Could you check a few things on this model? Use its own coordinates, in mm. Coordinates: 2 decimals unless noted, no trailing zeros.
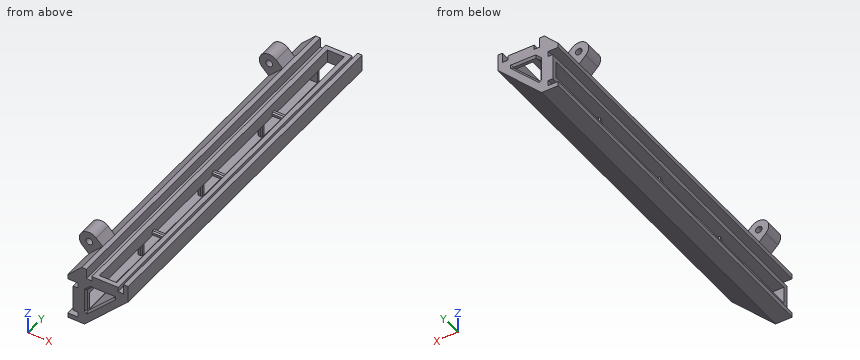
from build123d import *

# Parameters (mm, degrees)
BOSS_EXTRUDE4_DEPTH      = 247.65
CUT_EXTRUDE9_DEPTH       = 247.65
SKETCH11_W               = 11.65
SKETCH11_H               = 241.3
CUT_EXTRUDE7_DEPTH       = 9.017
SKETCH12_W               = 11.65
SKETCH12_H               = 241.3
CUT_EXTRUDE8_DEPTH       = 9.017
SKETCH16_R               = 2.286
BOSS_EXTRUDE5_DEPTH      = 12.7
CHAMFER1_SIZE            = 0.493914087
CHAMFER1_SIZE_2          = 0.6985
CHAMFER2_SIZE            = 3.175
CHAMFER3_SIZE            = 1.27
BOSS_EXTRUDE6_DEPTH      = 1.5875
BOSS_EXTRUDE6_DEPTH_BACK = 1.5875
SKETCH19_W               = 11.65
SKETCH19_H               = 3.175
SKETCH19_W_2             = 3.175
SKETCH19_H_2             = 11.4765
SKETCH20_W               = 3.175
SKETCH20_H               = 11.4765
SKETCH20_W_2             = 11.65
SKETCH20_H_2             = 3.175
BOSS_EXTRUDE7_DEPTH      = 3.175
CHAMFER4_SIZE            = 0.79375


with BuildPart() as part:
    # Sketch1 → Boss-Extrude4 (new body)
    with BuildSketch(Plane(origin=(0, 0, 0), x_dir=(1, 0, 0), z_dir=(0, 1, 0))):
        Polygon((41.275, 0), (41.275, 11.384871939), (11.384871939, 41.275), (0, 41.275), (0, 38.1), (6.858, 38.1), (6.858, 34.4), (3.683, 34.4), (3.683, 16.4), (6.858, 16.4), (6.858, 12.7), (0, 12.7), (0, 9.525), (9.525, 0), (12.7, 0), (12.7, 6.858), (16.4, 6.858), (16.4, 3.683), (34.4, 3.683), (34.4, 6.858), (38.1, 6.858), (38.1, 0), align=None)
    extrude(amount=BOSS_EXTRUDE4_DEPTH)

    # Sketch13 → Cut-Extrude9 (cut)
    with BuildSketch(Plane.XZ):
        Polygon((12.7, -12.7), (12.7, -31.75), (31.75, -12.7), align=None)
    extrude(amount=-CUT_EXTRUDE9_DEPTH, mode=Mode.SUBTRACT)

    # Sketch11 → Cut-Extrude7 (cut)
    with BuildSketch(Plane.ZY.offset(-3.683)):
        with Locations((-25.4, 123.825)):
            Rectangle(SKETCH11_W, SKETCH11_H)
    extrude(amount=-CUT_EXTRUDE7_DEPTH, mode=Mode.SUBTRACT)

    # Sketch12 → Cut-Extrude8 (cut)
    with BuildSketch(Plane.XY.offset(-3.683)):
        with Locations((25.4, 123.825)):
            Rectangle(SKETCH12_W, SKETCH12_H)
    extrude(amount=-CUT_EXTRUDE8_DEPTH, mode=Mode.SUBTRACT)

    # Sketch16 → Boss-Extrude5 (add)
    with BuildSketch(Plane(origin=(0, 225.425, 0), x_dir=(1, 0, 0), z_dir=(0, 1, 0))):
        with BuildLine():
            Line((5.034871939, -4.490128061), (9.525, 0))
            Line((9.525, 0), (0, 9.525))
            Line((0, 9.525), (-4.490128061, 5.034871939))
            ThreePointArc((-4.490128061, 5.034871939), (-4.490128061, -4.490128061), (5.034871939, -4.490128061))
        make_face()
        with Locations(Location((0.272371939, 0.272371939, 0), (0, 0, 270))):
            Circle(SKETCH16_R, mode=Mode.SUBTRACT)
    boss_extrude5 = extrude(amount=-BOSS_EXTRUDE5_DEPTH)

    # Mirror1: Boss-Extrude5 across plane
    add(boss_extrude5.mirror(Plane.ZX.offset(123.825)))

    # Chamfer1
    # the kernel refuses this chamfer: 0.6985, 0.493914087 mm, written as the material it adds along each edge
    with BuildSketch(Plane(origin=(31.75, 0, -12.7), x_dir=(-0.9984038297885895, 0, 0.056478249472492296), z_dir=(0, 1, 0))) as chamfer1_piece_1:
        Polygon((CHAMFER1_SIZE * 0.998403829099, -CHAMFER1_SIZE * 0.0564782494335), (CHAMFER1_SIZE_2 * 0.666041965215, -CHAMFER1_SIZE_2 * 0.745914271598), (0, 0), align=None)
    extrude(amount=247.65)
    with BuildSketch(Plane(origin=(12.7, 0, -31.75), x_dir=(0.745914271597676, 0, 0.6660419652145867), z_dir=(0, 1, 0))) as chamfer1_piece_2_section:
        Polygon((CHAMFER1_SIZE * 0.998403829099, -CHAMFER1_SIZE * 0.0564782494335), (CHAMFER1_SIZE_2 * 0.666041965215, -CHAMFER1_SIZE_2 * 0.745914271598), (0, 0), align=None)
    chamfer1_piece_2 = extrude(amount=247.65, mode=Mode.PRIVATE)
    chamfer1_piece_2 = split(chamfer1_piece_2, bisect_by=Plane(origin=(12.824663098, 1.5875, -31.225), z_dir=(0, 0, -1)), keep=Keep.TOP, mode=Mode.PRIVATE)
    add(chamfer1_piece_2)
    with BuildSketch(Plane(origin=(12.7, 0, -31.75), x_dir=(0.745914271597676, 0, 0.6660419652145867), z_dir=(0, 1, 0))) as chamfer1_piece_3_section:
        Polygon((CHAMFER1_SIZE * 0.998403829099, -CHAMFER1_SIZE * 0.0564782494335), (CHAMFER1_SIZE_2 * 0.666041965215, -CHAMFER1_SIZE_2 * 0.745914271598), (0, 0), align=None)
    chamfer1_piece_3 = extrude(amount=249.446320567, mode=Mode.PRIVATE)
    chamfer1_piece_3 = split(chamfer1_piece_3, bisect_by=Plane(origin=(12.757833333, 3.175, -31.167166667), z_dir=(0, -1, 0)), keep=Keep.TOP, mode=Mode.PRIVATE)
    add(chamfer1_piece_3)
    with BuildSketch(Plane(origin=(12.7, -1.796320567, -31.75), x_dir=(0.745914271597676, 0, 0.6660419652145867), z_dir=(0, 1, 0))) as chamfer1_piece_4_section:
        Polygon((CHAMFER1_SIZE * 0.998403829099, -CHAMFER1_SIZE * 0.0564782494335), (CHAMFER1_SIZE_2 * 0.666041965215, -CHAMFER1_SIZE_2 * 0.745914271598), (0, 0), align=None)
    chamfer1_piece_4 = extrude(amount=249.446320567, mode=Mode.PRIVATE)
    chamfer1_piece_4 = split(chamfer1_piece_4, bisect_by=Plane(origin=(12.757833333, 244.475, -31.167166667), z_dir=(0, 1, 0)), keep=Keep.TOP, mode=Mode.PRIVATE)
    add(chamfer1_piece_4)

    # Chamfer2
    chamfer2_edges = [part.edges().sort_by_distance(p)[0] for p in [
        (12.7, 123.825, -12.7),
    ]]
    chamfer(chamfer2_edges, length=CHAMFER2_SIZE)

    # Chamfer3
    chamfer3_edges = [part.edges().sort_by_distance(p)[0] for p in [
        (22.152667957, 0, -22.297332043),
        (22.152667957, 247.65, -22.297332043),
        (23.565542957, 0, -12.7),
        (23.565542957, 247.65, -12.7),
        (12.874625, 0, -31.226125),
        (12.874625, 247.65, -31.226125),
        (31.256085913, 0, -12.946957043),
        (31.256085913, 247.65, -12.946957043),
        (12.7, 0, -23.46325),
        (12.7, 247.65, -23.46325),
        (14.2875, 0, -14.2875),
        (14.2875, 247.65, -14.2875),
    ]]
    chamfer(chamfer3_edges, length=CHAMFER3_SIZE)

    # Sketch19 → Boss-Extrude6 (add, two sides: drawn at the far end of the back side and taken through both)
    with BuildSketch(Plane(origin=(0, 123.825, 0), x_dir=(1, 0, 0), z_dir=(0, 1, 0)).offset(-BOSS_EXTRUDE6_DEPTH_BACK)):
        with Locations((25.4, 11.1125)):
            Rectangle(SKETCH19_W, SKETCH19_H)
        with Locations((11.1125, 25.31325)):
            Rectangle(SKETCH19_W_2, SKETCH19_H_2)
    extrude(amount=BOSS_EXTRUDE6_DEPTH + BOSS_EXTRUDE6_DEPTH_BACK)

    # Sketch20 → Boss-Extrude7 (add)
    with BuildSketch(Plane(origin=(0, 185.7375, 0), x_dir=(1, 0, 0), z_dir=(0, 1, 0))):
        with Locations((11.1125, 25.31325)):
            Rectangle(SKETCH20_W, SKETCH20_H)
        with Locations((25.4, 11.1125)):
            Rectangle(SKETCH20_W_2, SKETCH20_H_2)
    boss_extrude7 = extrude(amount=BOSS_EXTRUDE7_DEPTH)

    # Mirror2: Boss-Extrude7 across plane
    add(boss_extrude7.mirror(Plane.ZX.offset(123.825)))

    # Chamfer4
    chamfer4_edges = [part.edges().sort_by_distance(p)[0] for p in [
        (25.4, 122.2375, -12.7),
        (25.4, 122.2375, -9.525),
        (25.4, 125.4125, -9.525),
        (25.4, 125.4125, -12.7),
        (9.525, 122.2375, -25.31325),
        (12.7, 122.2375, -25.31325),
        (12.7, 125.4125, -25.31325),
        (9.525, 125.4125, -25.31325),
        (9.525, 185.7375, -25.31325),
        (12.7, 185.7375, -25.31325),
        (9.525, 188.9125, -25.31325),
        (12.7, 188.9125, -25.31325),
        (25.4, 185.7375, -12.7),
        (25.4, 185.7375, -9.525),
        (25.4, 188.9125, -12.7),
        (25.4, 188.9125, -9.525),
        (9.525, 58.7375, -25.31325),
        (12.7, 58.7375, -25.31325),
        (9.525, 61.9125, -25.31325),
        (12.7, 61.9125, -25.31325),
        (25.4, 58.7375, -12.7),
        (25.4, 58.7375, -9.525),
        (25.4, 61.9125, -12.7),
        (25.4, 61.9125, -9.525),
    ]]
    chamfer(chamfer4_edges, length=CHAMFER4_SIZE)


solid = part.part
1) Imagine slicing it at A-A on y = 221. State how many separate pieces and enclosed holes the cut face has, plus the area to 3 significant figures.
2) Will these pins go through, and if not, where does the flat tip stop? pin 1 (1 mm diameter, centred on y = 137, z = -11, fed in from -X); pin 2 (2 mm diameter, centred on x = 26.5, y = 154, fed in from +Z); pin 3 (4 mm diameter, centred on x = 32.5, y = 58, fed in from +Z).
3) If I drill on L1, parallel to X at y = 34.5, z = -10.5 (3 decimals); L2, parallel to X at y = 104, z = -4 (3 decimals); L3, parallel to X at y = 178, z = -1 (3 decimals), over which ranges is the centre line in solid material (lowest first)?
Solved:
1. separate pieces: 2
1. enclosed holes: 1
1. area: 732 mm2
2. pin 1: stops at x = 0
2. pin 2: stops at z = -16.95
2. pin 3: stops at z = -3.68
3. L1: x = 0 to 19.575, 31.225 to 41.275
3. L2: x = 5.525 to 12.7, 16.4 to 19.575, 31.225 to 34.4, 38.1 to 41.275
3. L3: x = 8.525 to 12.7, 38.1 to 41.275
